The listing builds one solid part. Answer for the finished solid, in the listing's coordinates (mm). A direction names the side the tool comes from. Coordinates: 2 decimals unless noted, no trailing zeros. Loops run counter-clockwise (first coordinate to the right, second up) from the corner with the lowest first, then second, coordinate; pieces in that order, holes last. Notation, with made-up numbers: M 25,71 L 70,71 A25 cw 70,89 Z; hole C -23.5,-1.5 d4. An arc over 180 degrees is marked long. Return JSON: item names as keys, results as strings. Group by question number.
1. Section C-C (y = 49.5) is taken. Write down the section's boundary in (x, z) (3 decimals), then the cut area to 3 significant figures.
2. Which of the six approach directions +Z, -Z, +X, -X, +Y, -Y give full straight-line access (tool end or side, diameter ignored) to faces 5 (the face through (41.275, -1, 12)), 6 (the face through (39, -25.4, 54)), 7 (the face through (22.225, 17, 28))?
3. The mould has two halves that part along X. Classify faces 1 (the face through (-41.275, -1, 0)), 2 (the face through (45.8, -0.36, 57.15)), 3 (the face through (-4, 7.938, 38)), 4 (the face through (60, 2, 61.925)): pulls with the +X half, pulls with the -X half, needs draft (parallel to the pull), parting line crosses it, or undercut.
4. Section B-B (y = 22.5) is taken. Write down the section's boundary in (x, z) (3 decimals), then the cut area to 3 significant figures.
5. Straight lines are drawn through the part: L1, parallel to X at y = 29.5, z = 4 (3 decimals); L2, parallel to Z at x = 3, y = 54 (3 decimals); L3, parallel to Y at x = 1, z = 33.5. For each, find the intervals that lie inside material, in ascending order. Write a range as from..to.
6. Given P1, Ø10, axis at y = -21, z = 1.5, coming from the +X side (3 decimals); P2, Ø1.5, axis at x = 93, z = 65, coming from the -Y side; P3, Ø5, axis at y = 18, z = 23, coming from the -X side (3 decimals), each flat-ended and moving along its own axis, determine where each tip first touches the part or whether it passes through.
7. Section A-A (x = 78.5) is taken. Write down the section's boundary in (y, z) (3 decimals).
```python
from build123d import *

# Parameters (mm, degrees)
F1_DEPTH = 63.5
F0_W     = 25.3889229774
F0_H     = 19.05
F2_DEPTH = 25.4
F3_DEPTH = 7.9375
F5_R     = 6.35


with BuildPart() as f1:
    # F0 (on Front) → F1 (new body, symmetric)
    with BuildSketch(Plane.XZ):
        Polygon((41.275, -9.525), (41.275, 9.525), (22.225, 9.525), (-41.275, 9.525), (-41.275, -9.525), align=None)
    extrude(amount=F1_DEPTH, both=True)

    # F0 (on Front) → F2 (join, symmetric)
    with BuildSketch(Plane.XZ):
        with Locations((73.0194614887, 71.4502)):
            Rectangle(F0_W, F0_H)
        with BuildLine():
            Line((22.225, 9.525), (41.275, 9.525))
            Line((41.275, 9.525), (41.275, 46.0502))
            ThreePointArc((41.275, 46.0502), (45.9246798487, 57.2755201513), (57.15, 61.9252))
            Line((57.15, 61.9252), (60.325, 61.9252))
            Line((60.325, 61.9252), (60.325, 80.9752))
            Line((60.325, 80.9752), (57.15, 80.9752))
            ThreePointArc((57.15, 80.9752), (32.4542956671, 70.7459043329), (22.225, 46.0502))
            Line((22.225, 46.0502), (22.225, 9.525))
        make_face()
    extrude(amount=F2_DEPTH, both=True)

    # F0 (on Front) → F3 (join, symmetric)
    with BuildSketch(Plane.XZ):
        with BuildLine():
            Line((-41.275, 9.525), (22.225, 9.525))
            Line((22.225, 9.525), (22.225, 46.0502))
            ThreePointArc((22.225, 46.0502), (32.4542956671, 70.7459043329), (57.15, 80.9752))
            add(Edge.make_bspline(
                [(-41.275, 9.525), (-41.4512120187, 35.7986353338), (14.2870573327, 81.0561999679), (57.15, 80.9752)],
                knots=[0, 0, 0, 0, 121.6248811101, 121.6248811101, 121.6248811101, 121.6248811101], degree=3))
        make_face()
    extrude(amount=F3_DEPTH, both=True)

    # F0 (on Front) → F4 (revolve)
    with BuildSketch(Plane.XZ):
        Polygon((85.7139229774, 80.9752), (85.7139229774, 61.9252), (85.7139229774, 57.15), (111.125, 57.15), (111.125, 85.725), (85.7139229774, 85.725), align=None)
    revolve(axis=Axis((85.7139229774, 0, 71.4375), (0, 0, -1)))

    # F5
    f5_edges = [f1.edges().sort_by_distance(p)[0] for p in [
        (41.275, -63.5, 0),
        (-41.275, -63.5, 0),
        (-41.275, 63.5, 0),
        (41.275, 63.5, 0),
    ]]
    fillet(f5_edges, radius=F5_R)


solid = f1.part
```
Worked out:
{
 "1": {"outline": "M -41.275,-9.525 L 41.275,-9.525 L 41.275,9.525 L -41.275,9.525 Z", "area": "1,570 mm^2"},
 "2": {"face 5": "-Z, +X, +Y, -Y", "face 6": "+Z, +X, -X, -Y", "face 7": "+Z, -X, +Y"},
 "3": {"face 1": "pulls with the -X half", "face 2": "undercut", "face 3": "needs draft", "face 4": "undercut"},
 "4": {"outline": "M -41.275,-9.525 L 41.275,-9.525 L 41.275,46.05 A15.875 cw 57.15,61.925 L 73.904,61.925 L 73.904,57.15 L 97.524,57.15 L 97.524,85.725 L 73.904,85.725 L 73.904,80.975 L 57.15,80.975 A34.925 ccw 22.225,46.05 L 22.225,9.525 L -41.275,9.525 Z", "area": "4,020 mm^2"},
 "5": {"L1": "-41.275..41.275", "L2": "-9.525..9.525", "L3": "-7.94..7.94"},
 "6": {"P1": "x = 41.275", "P2": "y = -24.56", "P3": "x = 22.225"},
 "7": {"outline": "M -25.4,61.925 L -24.366,61.925 L -24.366,57.15 L 24.366,57.15 L 24.366,61.925 L 25.4,61.925 L 25.4,80.975 L 24.366,80.975 L 24.366,85.725 L -24.366,85.725 L -24.366,80.975 L -25.4,80.975 Z"}
}
